Autodesk Inventor part; units mm, degrees
ref_plane "YZ Plane" through (0, 0, 0) normal (1, 0, 0) x (0, 1, 0)
ref_plane "XZ Plane" through (0, 0, 0) normal (0, 1, 0) x (-1, 0, 0)
ref_plane "XY Plane" through (0, 0, 0) normal (0, 0, 1) x (1, 0, 0)
sketch "Sketch1" plane through (0, 0, 0) normal (0, 1, 0) x (-1, 0, 0)
  line L0 (-7, 32) -> (7, 32)
  line L1 (7, 32) -> (7, -32)
  line L2 (7, -32) -> (-7, -32)
  line L3 (-7, -32) -> (-7, 32)
  line L4 (-7, 32) -> (7, -32) construction
  line L5 (7, 32) -> (-7, -32) construction
  circle A0 centre (0, 25) radius 2.75
  circle A1 centre (0, -25) radius 2.75
  line L6 (0, 25) -> (0, 0) construction
  line L7 (0, 0) -> (0, -25) construction
  dimension "d0" = 5.5
  dimension "d1" = 50
  dimension "d3" = 7
  dimension "d4" = 7
extrude "Extrusion1" add sketch "Sketch1" along normal blind 7.4
sketch "Sketch2" plane through (7, 0, 32) normal (1, 0, 0) x (0, 0, -1)
  line L0 (64, 7.4) -> (0, 7.4) construction
  line L1 (14, 7.4) -> (24, 4)
  line L2 (24, 4) -> (32, 4)
  line L3 (32, 4) -> (32, 0) construction
  line L4 (50, 7.4) -> (40, 4)
  line L5 (40, 4) -> (32, 4)
  line L6 (14, 7.4) -> (50, 7.4)
  line L7 (0, 0) -> (64, 0)
  line L8 (4.25, 7.4) -> (9.75, 7.4)
  point P0 (7, 7.4)
  dimension "d7" = 4
  dimension "d8" = 7
  dimension "d9" = 10
extrude "Extrusion2" cut sketch "Sketch2" against normal through all
fillet "Fillet1" radius 7 4 edges at (7, 3.7, 32) (-7, 3.7, 32) (-7, 3.7, -32) (7, 3.7, -32)
properties part number "CH_01_0052_bracket_mount"
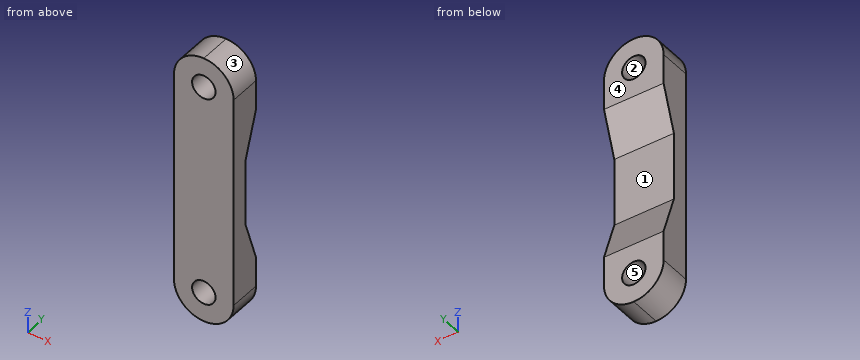
Geometry check sheet. Reference: the model listing, model coordinates, mm. Face numbers are marked on the shaded views. A direction names the side the tool comes from. Coordinates: 2 decimals unless noted, no trailing zeros. Order: outer loops, then holes, each group sorted by start corner. A loop starts at its lowest first (then second) coordinate and runs counter-clockwise, first axis right, second up. Notation, with made-up numbers: (16, -34) -> (28, -34) arc R20 cw to (28, -7) -> close; hole circle Ø5 at (7, 58). An arc over 180 degrees is marked (long way). Use a Markdown table: item, result. Add a question column.
1. Mould release check, pull along Z, two halves, no side actions. Record for the marked faces 3, 4 and 5: pulls with the +Z half, pulls with the -Z half, needs draft (parallel to the pull), parting line crosses it, or undercut.
2. Go/stop test with a flat-tipped pin: pin 1 Ø3.5 at (x, z) = (0, -25) entering from -Y. Record where the tip stops, or that it passes through.
3. Cross-section at C-C (z = -14.5). Enter the section's corners in (x, y), and give its area (3 significant figures).
4. Set-up check for the marked faces 1 and 2: record each of +Z, -Z, +X, -X, +Y, -Y from which the full face is reachable in a straight line by a thin tool's end or side.
5. Material ranges on L1, parallel to Z at x = 0, y = 1.5; L2, parallel to Z at x = -2.25, y = 2; L3, parallel to Y at x = -4, z = 8, recorded low to high.
6. Cross-section at D-D (z = 6.5). Enter the section's corners in (x, y), and give its area (3 significant figures).
7. Cross-section at A-A (y = 5). Give the number of separate pieces and of enclosed holes in the cut face, and give its area (3 significant figures).
8. Cross-section at B-B (x = -5). Enter the section's corners in (y, z).
Filled sheet:
| question | item | result |
|---|---|---|
| 1 | face 3 | pulls with the +Z half |
| 1 | face 4 | needs draft |
| 1 | face 5 | undercut |
| 2 | pin 1 | through |
| 3 | outline | (-7, 0) -> (7, 0) -> (7, 6.21) -> (-7, 6.21) -> close |
| 3 | area | 86.9 mm2 |
| 4 | face 1 | +X, -X, +Y |
| 4 | face 2 | +Y, -Y |
| 5 | L1 | -32 to -27.75, -22.25 to 22.25, 27.75 to 32 |
| 5 | L2 | -31.63 to -26.58, -23.42 to 23.42, 26.58 to 31.63 |
| 5 | L3 | 0 to 4 |
| 6 | outline | (-7, 0) -> (7, 0) -> (7, 4) -> (-7, 4) -> close |
| 6 | area | 56.0 mm2 |
| 7 | separate pieces | 2 |
| 7 | enclosed holes | 2 |
| 7 | area | 500 mm2 |
| 8 | outline | (0, -29.9) -> (7.4, -29.9) -> (7.4, -18) -> (4, -8) -> (4, 8) -> (7.4, 18) -> (7.4, 29.9) -> (0, 29.9) -> close |
